Geometry check sheet. Reference: the model listing, model coordinates, mm. Give positions to 0.01 mm unless a question says otherwise; leave off trailing zeros. Loops run counter-clockwise (first coordinate to the right, second up) from the corner with the lowest first, then second, coordinate; pieces in that order, holes last. Notation, with made-up numbers: (83, 48.25) -> (114, 48.25) arc R20 ccw to (114, 70.25) -> close; hole circle Ø1 at (69, -15). An arc over 180 degrees is marked (long way). Answer in a Markdown table with one row per item. Add a question column.
```python
from build123d import *

# Parameters (mm, degrees)
SKETCH1_R           = 1.7
BOSS_EXTRUDE1_DEPTH = 8
FILLET1_R           = 10
SKETCH2_R           = 1.7
CUT_EXTRUDE1_DEPTH  = 39


with BuildPart() as part:
    # Sketch1 → Boss-Extrude1 (new body)
    with BuildSketch(Plane(origin=(0, 0, 0), x_dir=(1, 0, 0), z_dir=(0, 1, 0))):
        with BuildLine():
            ThreePointArc((-5.409133759, 74.8046875), (-53.033008589, 53.033008589), (-74.8046875, 5.409133759))
            ThreePointArc((-74.8046875, 5.409133759), (-87.5, 0), (-74.8046875, -5.409133759))
            ThreePointArc((-74.8046875, -5.409133759), (-53.033008589, -53.033008589), (-5.409133759, -74.8046875))
            ThreePointArc((-5.409133759, -74.8046875), (0, -87.5), (5.409133759, -74.8046875))
            ThreePointArc((5.409133759, -74.8046875), (53.033008589, -53.033008589), (74.8046875, -5.409133759))
            ThreePointArc((74.8046875, -5.409133759), (87.5, 0), (74.8046875, 5.409133759))
            ThreePointArc((74.8046875, 5.409133759), (53.033008589, 53.033008589), (5.409133759, 74.8046875))
            ThreePointArc((5.409133759, 74.8046875), (0, 87.5), (-5.409133759, 74.8046875))
        make_face()
        with Locations(Location((-80, 0, 0), (0, 0, 270))):
            Circle(SKETCH1_R, mode=Mode.SUBTRACT)
        with Locations(Location((80, 0, 0), (0, 0, 270))):
            Circle(SKETCH1_R, mode=Mode.SUBTRACT)
        with Locations(Location((0, 80, 0), (0, 0, 270))):
            Circle(SKETCH1_R, mode=Mode.SUBTRACT)
        with Locations(Location((0, -80, 0), (0, 0, 270))):
            Circle(SKETCH1_R, mode=Mode.SUBTRACT)
    extrude(amount=BOSS_EXTRUDE1_DEPTH)

    # Fillet1
    fillet1_edges = [part.edges().sort_by_distance(p)[0] for p in [
        (74.8046875, 4, -5.409133759),
        (74.8046875, 4, 5.409133759),
        (5.409133759, 4, 74.8046875),
        (-5.409133759, 4, 74.8046875),
        (-74.8046875, 4, 5.409133759),
        (-74.8046875, 4, -5.409133759),
        (-5.409133759, 4, -74.8046875),
        (5.409133759, 4, -74.8046875),
    ]]
    fillet(fillet1_edges, radius=FILLET1_R)

    # Sketch2 → Cut-Extrude1 (cut)
    with BuildSketch(Plane(origin=(0, 8, 0), x_dir=(1, 0, 0), z_dir=(0, 1, 0))):
        with Locations(Location((0, 38, 0), (0, 0, 270))):
            Circle(SKETCH2_R)
        with Locations(Location((32.908965344, -19, 0), (0, 0, 270))):
            Circle(SKETCH2_R)
        with Locations(Location((-32.908965344, -19, 0), (0, 0, 270))):
            Circle(SKETCH2_R)
    extrude(amount=-CUT_EXTRUDE1_DEPTH, mode=Mode.SUBTRACT)


solid = part.part
```
1. Sectioned sample at B-B (x = 25.5). Enter the section's corners in (y, z), plus the area to 3 significant figures.
2. Gauge pin test, flat ends, axial feed: pin 1 Ø1.5 at (x, y) = (57.5, 5) entering from +Z; pin 2 Ø4 at (x, y) = (-53.5, 5.5) entering from +Z; pin 3 Ø1.5 at (x, y) = (-46.5, 2.5) entering from -Z. Record the tip position at first contact, or that the pin passes through.
3. Sectioned sample at A-A (z = -45.5). Enter the section's corners in (x, y).
4. Material ranges on L1, parallel to X at y = 4.75, z = 0; L2, parallel to X at y = 3, z = -38; L3, parallel to X at y = 4.5, z = 80, recorded low to high. Write a range as from..to.
5. Sectioned sample at C-C (y = 3). Count the separate pieces of the cut face and the enclosed holes in it, plus the area to 3 significant figures.
Response:
| question | item | result |
|---|---|---|
| 1 | outline | (0, -70.53) -> (8, -70.53) -> (8, 70.53) -> (0, 70.53) -> close |
| 1 | area | 1,130 mm2 |
| 2 | pin 1 | stops at z = 49.04 |
| 2 | pin 2 | stops at z = 54.52 |
| 2 | pin 3 | stops at z = -59.43 |
| 3 | outline | (-59.62, 0) -> (59.62, 0) -> (59.62, 8) -> (-59.62, 8) -> close |
| 4 | L1 | x = -87.5..-81.7, -78.3..78.3, 81.7..87.5 |
| 4 | L2 | x = -64.66..-1.7, 1.7..64.66 |
| 4 | L3 | x = -7.74..-1.7, 1.7..7.74 |
| 5 | separate pieces | 1 |
| 5 | enclosed holes | 7 |
| 5 | area | 18,400 mm2 |
